from build123d import *

# Parameters (mm, degrees)
BOSS_EXTRUDE9_DEPTH  = 35
SHELL1_T             = -2
SKETCH25_W           = 37
SKETCH25_H           = 30.5
CUT_EXTRUDE6_DEPTH   = 2
BOSS_EXTRUDE11_REACH = 61.969
CUT_EXTRUDE7_START   = -33
CUT_EXTRUDE7_DEPTH   = 27.688806668
BOSS_EXTRUDE12_DEPTH = 65
CUT_EXTRUDE9_START   = -1.04026
CUT_EXTRUDE9_DEPTH   = 1.04026
BOSS_EXTRUDE13_DEPTH = 4
CUT_EXTRUDE14_DEPTH  = 4


# Read off the part's stored shape, not the designer's step: Cut-Extrude7
with BuildPart() as part:
    # Sketch24 → Boss-Extrude9 (new, symmetric)
    with BuildSketch(Plane(origin=(0, 0, 0), x_dir=(0, 0, -1), z_dir=(1, 0, 0))):
        Polygon((0, 0), (5, 35), (14.77647195, 35), (33.857142857, 20), (33.857142857, 13.020408163), align=None)
    extrude(amount=BOSS_EXTRUDE9_DEPTH, both=True)

    # Shell1
    shell1_openings = [part.faces().sort_by_distance(p)[0] for p in [
        (0, 6.510204082, -16.928571429),
    ]]
    offset(amount=SHELL1_T, openings=shell1_openings, kind=Kind.INTERSECTION)

    # Sketch25 → Cut-Extrude6 (cut)
    with BuildSketch(Plane(origin=(0, 0, 0), x_dir=(1, 0, 0), z_dir=(0, 0.1414213562373094, 0.9899494936611667))):
        with Locations((13.5, 17.105339059)):
            Rectangle(SKETCH25_W, SKETCH25_H)
    extrude(amount=-CUT_EXTRUDE6_DEPTH, mode=Mode.SUBTRACT)

    # Boss-Extrude11: up to this plane
    boss_extrude11_end = Plane(origin=(35, 0, 0), z_dir=(0, 0.9333601055458265, 0.35894137874517024))
    # Sketch27 → Boss-Extrude11 (add, up to the surface)
    with BuildSketch(Plane(origin=(0, 35, 0), x_dir=(1, 0, 0), z_dir=(0, 1, 0)), mode=Mode.PRIVATE) as boss_extrude11_sk1:
        Polygon((-5.311193332, 5), (-19.86581292, -5.902882273), (-35, -5.902882273), (-35, 5), align=None)
    boss_extrude11_tool1 = split(extrude(boss_extrude11_sk1.sketch, amount=-BOSS_EXTRUDE11_REACH, mode=Mode.PRIVATE), bisect_by=boss_extrude11_end, keep=Keep.BOTH, mode=Mode.PRIVATE)
    add(boss_extrude11_tool1.solids().sort_by_distance((-23.400412, 35, -0.138611))[0])

    # Cut-Extrude7 outline → Cut-Extrude7 (cut)
    with BuildSketch(Plane.YZ.offset(CUT_EXTRUDE7_START)):
        Polygon((20.857864376, -5), (1.922845087, -2.294997245), (1.922845087, -5), align=None)
    extrude(amount=CUT_EXTRUDE7_DEPTH, mode=Mode.SUBTRACT)

    # Sketch30 → Boss-Extrude12 (add)
    with BuildSketch(Plane.ZY.offset(35)):
        Polygon((-33.857142857, 20), (-33.857142857, 13.020408163), (5.902882273, -2.270065636), (5.902882273, 35), (-14.77647195, 35), align=None)
    extrude(amount=BOSS_EXTRUDE12_DEPTH)

    # Sketch31 → Cut-Extrude9 (cut)
    with BuildSketch(Plane(origin=(0, 1.922845087, 0), x_dir=(1, 0, 0), z_dir=(0, 1, 0)).offset(CUT_EXTRUDE9_START)):
        Polygon((-8.922191333, 2.294997244), (-5.311193332, 5), (-33, 5), (-33, 2.294997244), align=None)
    extrude(amount=CUT_EXTRUDE9_DEPTH, mode=Mode.SUBTRACT)

    # Sketch26 → Boss-Extrude13 (add)
    with BuildSketch(Plane(origin=(35, 0, 0), x_dir=(0, 0, -1), z_dir=(1, 0, 0))):
        Polygon((5, 35), (0, 0), (33.857142857, 13.020408163), (33.857142857, 20), (14.77647195, 35), align=None)
    extrude(amount=BOSS_EXTRUDE13_DEPTH)

    # Sketch36 → Cut-Extrude14 (cut)
    with BuildSketch(Plane.ZY.offset(-33)):
        Polygon((-31.857142857, 12.251270128), (-2.137749704, 0.822112303), (-6.734590803, 33), (-14.084453997, 33), (-31.857142857, 19.028251617), align=None)
    extrude(amount=-CUT_EXTRUDE14_DEPTH, mode=Mode.SUBTRACT)


solid = part.part
Can you work these out from the model? Positions are in its coordinate system, mm. A direction names the side the tool comes from. Round coordinates to 2 decimals unless told otherwise and drop trailing zeros. Loops run counter-clockwise (first coordinate to the right, second up) from the corner with the lowest first, then second, coordinate; pieces in that order, holes last. Notation, with made-up numbers: (74.25, -29.5) - (91.25, -29.5) arc R26 cw to (91.25, -2.5) - close; hole circle Ø6 at (72.5, 61). An arc over 180 degrees is marked (long way). Write item = value, one per line. Start each with the question number.
(1) If we mould it in two halves opening along Z, with no side actions, what happens to faces 1 (the face through (32.27, 17.58, -2.51)), 2 (the face through (-33, 17, -14)), 3 (the face through (2, 33, -10)), 4 (the face through (-5, 17, -3))? For each: released by +Z, released by -Z, zero draft, split by the parting line, or undercut.
(2) For P1, Ø2, axis at x = 7, z = -27.5, coming from the +Y side; P2, Ø3.5, axis at x = -4, z = -11, coming from the -Y side; P3, Ø7, axis at y = 23, z = -3, coming from the +X side; P4, Ø10, axis at x = -13, z = -24, coming from the +Y side, each with a flat end and sliding along its axis, tell me the tip position at first contact or that it passes through.
(3) If we section it at B-B (y = 10): Please give me the cut outline in (x, z), and give its area (3 significant figures).
(4) If I drill on probe 1 along X at (y, z) = (24, -9.5); probe 2 along Z at (x, y) = (-39, 31); probe 3 along Z at (x, y) = (-13.5, 29), over which ranges is the centre line in solid material (lowest first)? Write a range as [from, to].
(5) If we section it at A-A (x = 29): Please give me the cut outline in (y, z), and give its area (3 significant figures).
(6) If we section it at D-D (x = -31.5): Please give me the cut outline in (y, z) (3 decimals), and give its area (3 significant figures).
(7) If we section it at C-C (z = -26): Please give me the cut outline in (x, y).
(8) For faces 5 (the face through (32, 17, -3)), 6 (the face through (-14.104, 16.626, 1.587)), 7 (the face through (2, 16, -31.857)), which set-ups out of +Z, -Z, +X, -X, +Y, -Y let a thin tool reach every point of the face, with its end or its side?
Ans:
q1.face_1 = released by +Z
q1.face_2 = undercut
q1.face_3 = undercut
q1.face_4 = zero draft
q2.P1 = 25.78
q2.P2 = 33
q2.P3 = 39
q2.P4 = 31.68
q3.outline = (-100, -26) - (-33, -26) - (-33, -3.45) - (-5, -3.45) - (-5, -1.43) - (-10.08, -1.43) - (-19.87, 5.9) - (-100, 5.9) - close; (32, -3.45) - (37, -3.45) - (37, -26) - (39, -26) - (39, -1.43) - (32, -1.43) - close
q3.area = 2,390 mm²
q4.probe_1 = [-100, -33], [37, 39]
q4.probe_2 = [-19.86, 5.9]
q4.probe_3 = [-22.41, -19.17], [-6.16, 1.13]
q5.outline = (0, 0) - (0.82, -2.14) - (1.55, -2.24) - (1.84, -0.26) - close; (12.25, -31.86) - (13.02, -33.86) - (20, -33.86) - (35, -14.78) - (35, -5) - (32.03, -4.58) - (31.75, -6.56) - (33, -6.73) - (33, -14.08) - (19.03, -31.86) - close
q5.area = 84.6 mm²
q6.outline = (-2.27, 5.903) - (0.883, -2.295) - (1.923, -2.295) - (33, -6.735) - (33, -14.084) - (19.028, -31.857) - (12.251, -31.857) - (13.02, -33.857) - (20, -33.857) - (35, -14.776) - (35, 5.903) - close
q6.area = 447 mm²
q7.outline = (-100, 10) - (-33, 10) - (-33, 23.63) - (37, 23.63) - (37, 10) - (39, 10) - (39, 26.18) - (-100, 26.18) - close
q8.face_5 = +Z
q8.face_6 = +Z, +X, +Y
q8.face_7 = -Y
